Geometry check sheet. Reference: the model listing, model coordinates, mm. A direction names the side the tool comes from. Give positions to 0.01 mm unless a question says otherwise; leave off trailing zeros. Order: outer loops, then holes, each group sorted by start corner. A loop starts at its lowest first (then second) coordinate and runs counter-clockwise, first axis right, second up.
from build123d import *

# Parameters (mm, degrees)
ESQUISSE1_W        = 37.7
ESQUISSE1_H        = 37.7
BOSS_EXTRU_1_DEPTH = 40


with BuildPart() as part:
    # Esquisse1 → Boss.-Extru.1 (new body)
    with BuildSketch(Plane(origin=(0, 0, 0), x_dir=(1, 0, 0), z_dir=(0, 1, 0))):
        Rectangle(ESQUISSE1_W, ESQUISSE1_H)
        Polygon((-10.1, 10.1), (-2.4, 10.1), (-2.4, 3.85), (2.4, 3.85), (2.4, 10.1), (10.1, 10.1), (10.1, 2.4), (3.85, 2.4), (3.85, -2.4), (10.1, -2.4), (10.1, -10.1), (2.4, -10.1), (2.4, -3.85), (-2.4, -3.85), (-2.4, -10.1), (-10.1, -10.1), (-10.1, -2.4), (-3.85, -2.4), (-3.85, 2.4), (-10.1, 2.4), align=None, mode=Mode.SUBTRACT)
    boss_extru_1 = extrude(amount=BOSS_EXTRU_1_DEPTH)


with BuildPart() as sym_trie1_1:
    # Symétrie1: Boss.-Extru.1 across plane
    add(boss_extru_1.mirror(Plane.XY))


with BuildPart() as part_1:
    add(part.part)

    # Symétrie1 united with what the copies to: union Symétrie1_1
    add(sym_trie1_1.part)


solid = part_1.part
Item 1: Scan lines: L1, parallel to Z at x = 5, y = 15.5; L2, parallel to Z at x = 1.5, y = 7. Record each from-to range of solid material in increasing order.
Reported:
L1: z = -18.85 to -10.1, -2.4 to 2.4, 10.1 to 18.85
L2: z = -18.85 to -3.85, 3.85 to 18.85
Item 2: Sectioned sample at C-C (y = 10). Enter the section's corners in (x, z), and give its area (3 significant figures).
Reported:
outline: (-18.85, -18.85) - (18.85, -18.85) - (18.85, 18.85) - (-18.85, 18.85) - close; hole (-10.1, -10.1) - (-2.4, -10.1) - (-2.4, -3.85) - (2.4, -3.85) - (2.4, -10.1) - (10.1, -10.1) - (10.1, -2.4) - (3.85, -2.4) - (3.85, 2.4) - (10.1, 2.4) - (10.1, 10.1) - (2.4, 10.1) - (2.4, 3.85) - (-2.4, 3.85) - (-2.4, 10.1) - (-10.1, 10.1) - (-10.1, 2.4) - (-3.85, 2.4) - (-3.85, -2.4) - (-10.1, -2.4) - close
area: 1,130 mm2
Item 3: Sectioned sample at B-B (x = -1.5). Enter the section's corners in (y, z), and give its area (3 significant figures).
Reported:
outline: (0, -18.85) - (40, -18.85) - (40, -3.85) - (0, -3.85) - close; (0, 3.85) - (40, 3.85) - (40, 18.85) - (0, 18.85) - close
area: 1,200 mm2
Item 4: Sectioned sample at D-D (z = 0). Enter the section's corners in (x, y).
Reported:
outline: (-18.85, 0) - (-3.85, 0) - (-3.85, 40) - (-18.85, 40) - close; (3.85, 0) - (18.85, 0) - (18.85, 40) - (3.85, 40) - close
Item 5: Draft check along Z on faces 1 (the flat face through (7, 20, 2.4)), 2 (the flat face through (18.85, 20, 0)), 3 (the flat face through (0, 20, 18.85)). Enter one of: released by +Z, released by -Z, zero draft, split by the parting line, or undercut.
Reported:
face 1: undercut
face 2: zero draft
face 3: released by +Z
Item 6: Sectioned sample at A-A (z = 4.5). Enter the section's corners in (x, y), and give its area (3 significant figures).
Reported:
outline: (-18.85, 0) - (-10.1, 0) - (-10.1, 40) - (-18.85, 40) - close; (-2.4, 0) - (2.4, 0) - (2.4, 40) - (-2.4, 40) - close; (10.1, 0) - (18.85, 0) - (18.85, 40) - (10.1, 40) - close
area: 892 mm2
Item 7: Set-up check for faces 4 (the flat face through (-0.3, 0, -4.5)), 5 (the flat face through (3.85, 20, 0)): record each of +Z, -Z, +X, -X, +Y, -Y from which the full face is reachable in a straight line by a thin tool's end or side.
Reported:
face 4: +Z, -Z, +X, -X, -Y
face 5: +Y, -Y
